from build123d import *

# Parameters (mm, degrees)
F1_DEPTH = 15


with BuildPart() as f1:
    # F0 (on Front) → F1 (new body)
    with BuildSketch(Plane.XZ):
        with BuildLine():
            Line((-12.25, 3), (-12.25, 0))
            Line((-12.25, 0), (-2.25, 0))
            ThreePointArc((-2.25, 0), (0, 4), (2.25, 0))
            Line((2.25, 0), (12.25, 0))
            Line((12.25, 0), (12.25, 3))
            Line((12.25, 3), (4.25, 3))
            ThreePointArc((4.25, 3), (0, 5.8), (-4.25, 3))
            Line((-4.25, 3), (-12.25, 3))
        make_face()
    extrude(amount=F1_DEPTH)


solid = f1.part
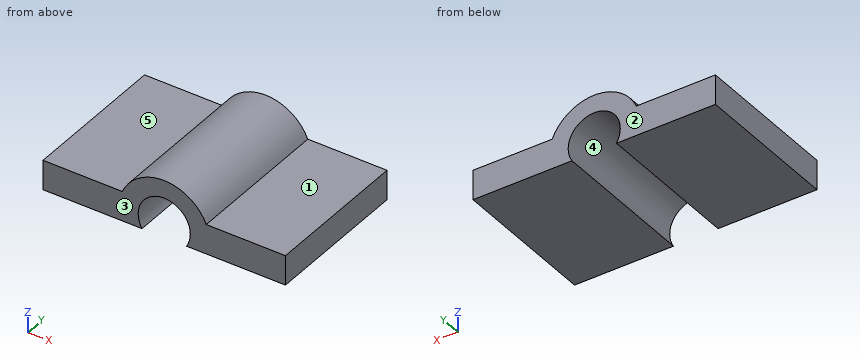
Read the model definition and answer for the solid it produces. Units are mm, in the model's axes. Face numbers are marked on the shaded views. A direction names the side the tool comes from. Round coordinates to 2 decimals unless told otherwise and drop trailing zeros. Write each loop counter-clockwise with the first axis right and the second up, starting at its lowest first coordinate (ties: lowest second). Pieces come first, ordered by that corner, then holes.
Q1. Straight lines are drawn through the part: line 1 (X direction, y = -10, z = 1.3); line 2 (Z direction, x = -10.25, y = -2.25); line 3 (X direction, y = -8.5, z = 3.45). For each, find the intervals that lie inside material, in ascending order.
Values:
line 1: x = -12.25 to -2.63, 2.63 to 12.25
line 2: z = 0 to 3
line 3: x = -4.03 to -1.61, 1.61 to 4.03
Q2. Find section D-D on z = 0.4. Determine the outline of the cut face in (x, y), and give its area (3 significant figures).
Values:
outline: (-12.25, -15) - (-2.45, -15) - (-2.45, 0) - (-12.25, 0) - close; (2.45, -15) - (12.25, -15) - (12.25, 0) - (2.45, 0) - close
area: 294 mm2
Q3. Find section C-C on x = 0. Determine the outline of the cut face in (y, z), and give its area (3 significant figures).
Values:
outline: (-15, 4) - (0, 4) - (0, 5.8) - (-15, 5.8) - close
area: 27.0 mm2
Q4. Find section B-B on z = 2.05. Determine the outline of the cut face in (x, y).
Values:
outline: (-12.25, -15) - (-2.54, -15) - (-2.54, 0) - (-12.25, 0) - close; (2.54, -15) - (12.25, -15) - (12.25, 0) - (2.54, 0) - close
Q5. A tool of negligible diameter and unlimited length cuts with its end or side. For the marked faces 1 and 2, from which of +Z, -Z, +X, -X, +Y, -Y can it reach the whole face along a straight path? Write none if from no direction.
Values:
face 1: +Z, +X, +Y, -Y
face 2: +Z, -Z, +X, -X, +Y
Q6. The mould has two halves that part along Z. Classify the marked faces 3, 4 and 5: released by +Z, released by -Z, zero draft, split by the parting line, or undercut.
Values:
face 3: zero draft
face 4: undercut
face 5: released by +Z
Q7. Flat-ended cylindrical pins translate along their axes: P1, Ø1, axis at x = -5, y = -10.5, coming from the +Z side; P2, Ø3, axis at x = 0, z = 1.37, coming from the +Y side. Find the tip coordinate at first contact, or state that the pin passes through.
Values:
P1: stops at z = 3
P2: passes through
Q8. Find section A-A on y = -10.25. Determine the outline of the cut face in (x, z), and give its area (3 significant figures).
Values:
outline: (-12.25, 0) - (-2.25, 0) arc R2.63 cw (long way) to (2.25, 0) - (12.25, 0) - (12.25, 3) - (4.25, 3) arc R4.63 ccw to (-4.25, 3) - (-12.25, 3) - close
area: 72.9 mm2
